```python
from build123d import *

# Parameters (mm, degrees)
SKETCH1_R           = 38.1
SKETCH1_R_2         = 3.302
BOSS_EXTRUDE1_DEPTH = 6.35
CUT_EXTRUDE4_DEPTH  = 55.254423783
CIRPATTERN1_COUNT   = 4


with BuildPart() as part:
    # Sketch1 → Boss-Extrude1 (new body)
    with BuildSketch(Plane(origin=(0, 0, 0), x_dir=(1, 0, 0), z_dir=(0, 1, 0))):
        with Locations(Location((0, 0, 0), (0, 0, 270))):
            Circle(SKETCH1_R)
        with Locations(Location((0, 0, 0), (0, 0, 270))):
            Circle(SKETCH1_R_2, mode=Mode.SUBTRACT)
    extrude(amount=BOSS_EXTRUDE1_DEPTH)

    # Sketch2 → Cut-Extrude4 (cut, through all)
    with BuildSketch(Plane(origin=(0, 0, 0), x_dir=(1, 0, 0), z_dir=(0, 1, 0))):
        with BuildLine():
            Line((-31.590851128, 3.175), (-9.114849368, 3.175))
            ThreePointArc((-9.114849368, 3.175), (-6.824994652, 6.824994652), (-3.175, 9.114849368))
            Line((-3.175, 9.114849368), (-3.175, 31.590851128))
            ThreePointArc((-3.175, 31.590851128), (-22.450640303, 22.450640303), (-31.590851128, 3.175))
        make_face()
    cut_extrude4 = extrude(amount=CUT_EXTRUDE4_DEPTH, mode=Mode.SUBTRACT)

    # CirPattern1: Cut-Extrude4 ×4 about axis
    cirpattern1_axis = Axis((0, 0, 0), (0, 1, 0))
    for i in range(1, CIRPATTERN1_COUNT):
        add(cut_extrude4.rotate(cirpattern1_axis, i * 360 / CIRPATTERN1_COUNT), mode=Mode.SUBTRACT)


solid = part.part
```
Work out the finished part from the listing and answer in its coordinate system (mm). Coordinates: 2 decimals unless noted, no trailing zeros. Write each loop counter-clockwise with the first axis right and the second up, starting at its lowest first coordinate (ties: lowest second). Pieces come first, ordered by that corner, then holes.
Q1. A cutting plane is placed at A-A, the plane z = 0. Give the vertices of the cut face in (x, y).
Q2. Find the intervals of material crossed by line 1 (X direction, y = 4.75, z = 0); line 2 (X direction, y = 3.5, z = -24) (3 decimals); line 3 (Z direction, x = 23, y = 5) (1 decimal), in increasing order.
Q3. Determine the mould class of faces 1 (the face through (1, 0, 8)), 2 (the face through (3.175, 3, -21)), 3 (the face through (-23.183, 3.131, -30.235)) for opening direction Z: released by +Z, released by -Z, zero draft, split by the parting line, or undercut.
Q4. A cutting plane is placed at D-D, the plane z = 24.5. Give the vertices of the cut face in (x, y) (3 decimals).
Q5. A cutting plane is placed at C-C, the plane x = 0. Give the vertices of the cut face in (y, z), then the cut area to 3 significant figures.
Q6. A cutting plane is placed at B-B, the plane y = 1.75. Give the vertices of the cut face in (x, z) (3 decimals).
Q7. Each of these flat-tipped pins is pushed along its axis until it touches: pin 1 Ø1.9 at (x, y) = (-22, 3) entering from +Z; pin 2 Ø1.5 at (x, y) = (-4.5, 4) entering from -Z (3 decimals); pin 3 Ø1.5 at (x, y) = (-18, 3) entering from -Z. Where does it stop, or does it pass through?
Findings below:
1. outline: (-38.1, 0) - (-3.3, 0) - (-3.3, 6.35) - (-38.1, 6.35) - close; (3.3, 0) - (38.1, 0) - (38.1, 6.35) - (3.3, 6.35) - close
2. line 1: x = -38.1 to -3.3, 3.3 to 38.1
2. line 2: x = -29.591 to -20.786, -3.175 to 3.175, 20.786 to 29.591
2. line 3: z = -30.4 to -21.9, -3.2 to 3.2, 21.9 to 30.4
3. face 1: zero draft
3. face 2: undercut
3. face 3: split by the parting line
4. outline: (-29.178, 0) - (-20.194, 0) - (-20.194, 6.35) - (-29.178, 6.35) - close; (-3.175, 0) - (3.175, 0) - (3.175, 6.35) - (-3.175, 6.35) - close; (20.194, 0) - (29.178, 0) - (29.178, 6.35) - (20.194, 6.35) - close
5. outline: (0, -38.1) - (6.35, -38.1) - (6.35, -3.3) - (0, -3.3) - close; (0, 3.3) - (6.35, 3.3) - (6.35, 38.1) - (0, 38.1) - close
5. area: 442 mm2
6. outline: circle Ø76.2 at (0, 0); hole (-31.591, -3.175) arc R31.75 ccw to (-3.175, -31.591) - (-3.175, -9.115) arc R9.652 cw to (-9.115, -3.175) - close; hole (-31.591, 3.175) - (-9.115, 3.175) arc R9.652 cw to (-3.175, 9.115) - (-3.175, 31.591) arc R31.75 ccw to start; hole circle Ø6.604 at (0, 0); hole (3.175, -31.591) arc R31.75 ccw to (31.591, -3.175) - (9.115, -3.175) arc R9.652 cw to (3.175, -9.115) - close; hole (3.175, 9.115) arc R9.652 cw to (9.115, 3.175) - (31.591, 3.175) arc R31.75 ccw to (3.175, 31.591) - close
7. pin 1: stops at z = 31.76
7. pin 2: stops at z = -37.915
7. pin 3: stops at z = -33.97
